Geometry check sheet. Reference: drawing and pictorial views, mm from the part's lowest x, y, z. A direction names the side the tool comes from. Give positions to 0.01 mm unless a question says otherwise; leave off trailing zeros. Loops run counter-clockwise (first coordinate to the right, second up) from the corner with the lowest first, then second, coordinate; pieces in that order, holes last. Notation, with made-up numbers: (76.5, -37.5) -> (94.5, -37.5) arc R25 cw to (94.5, 1.5) -> close; hole circle Ø7 at (86.25, 64). An arc over 180 degrees is marked (long way). Write item = value, one per line. Start each with the question number.
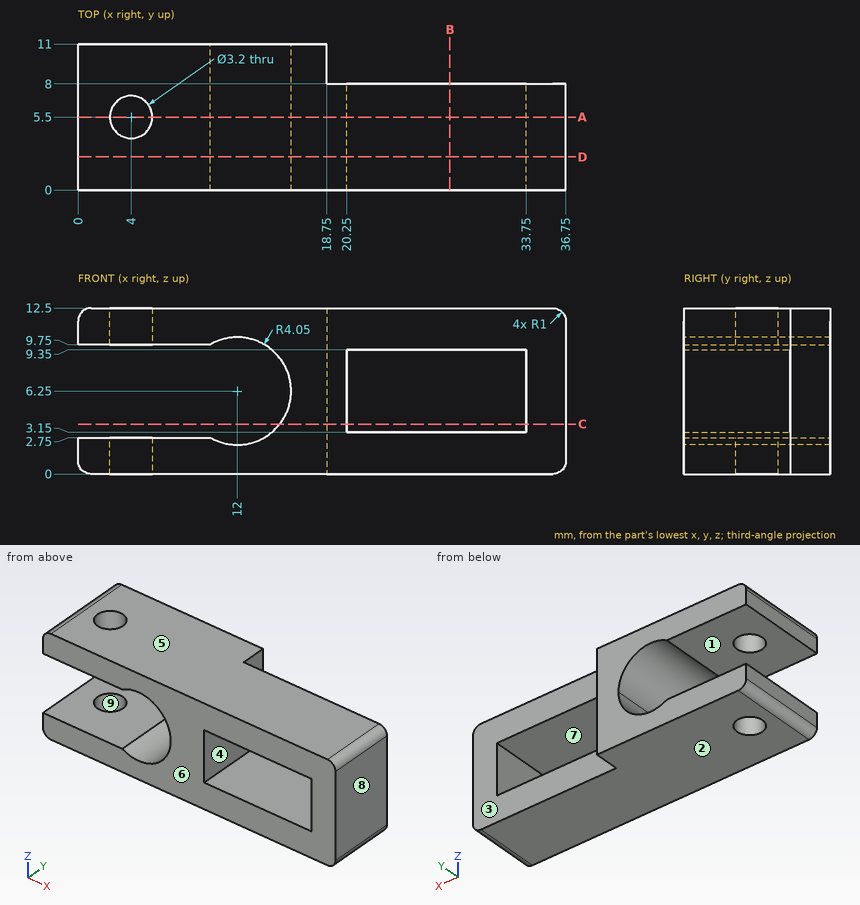
1) Draft check along X on the marked faces 6, 7, 8 and 9. Enter one of: released by +X, released by -X, zero draft, split by the parting line, or undercut.
2) Section check C-C (z = 3.75). Enter the section's corners in (x, y), plus the area to 3 significant figures.
3) Depth check by flat-ended pin: pin 1 Ø3 at (x, y) = (4, 5.5) entering from +Z; pin 2 Ø2.5 at (y, z) = (9.5, 3.5) entering from +X; pin 3 Ø3 at (y, z) = (3, 7) entering from -X. Enter the tip coordinate at first touch or a pass-through.
4) Thickness scan on line 1 (Y direction, x = 4, z = 11.5); line 2 (Z direction, x = 12, y = 8.5); line 3 (Z direction, x = 5, y = 2.75). Record the ranges inside material, lowest first.
5) Section check B-B (x = 28). Enter the section's corners in (y, z), plus the area to 3 significant figures.
6) Section check D-D (y = 2.5). Enter the section's corners in (x, z), plus the area to 3 significant figures.
7) Tool access check on the marked faces 1, 2, 3, 4 and 5. Record the directions out of +Z, -Z, +X, -X, +Y, -Y that give a thin tool (end or side, any length) a straight path to the whole face; none if there is none.
8) Section check A-A (y = 5.5). Enter the section's corners in (x, z).
Check result:
q1.face_6 = zero draft
q1.face_7 = undercut
q1.face_8 = released by +X
q1.face_9 = undercut
q2.outline = (15.19, 0) -> (20.25, 0) -> (20.25, 8) -> (18.75, 8) -> (18.75, 11) -> (15.19, 11) -> close; (33.75, 0) -> (36.75, 0) -> (36.75, 8) -> (33.75, 8) -> close
q2.area = 75.2 mm2
q3.pin_1 = through
q3.pin_2 = 18.75
q3.pin_3 = 15.37
q4.line_1 = 0 to 3.9, 7.1 to 11
q4.line_2 = 0 to 2.2, 10.3 to 12.5
q4.line_3 = 0 to 2.75, 9.75 to 12.5
q5.outline = (0, 0) -> (8, 0) -> (8, 3.15) -> (0, 3.15) -> close; (0, 9.35) -> (8, 9.35) -> (8, 12.5) -> (0, 12.5) -> close
q5.area = 50.4 mm2
q6.outline = (0, 1) arc R1 ccw to (1, 0) -> (35.75, 0) arc R1 ccw to (36.75, 1) -> (36.75, 11.5) arc R1 ccw to (35.75, 12.5) -> (1, 12.5) arc R1 ccw to (0, 11.5) -> (0, 9.75) -> (9.96, 9.75) arc R4.05 cw (long way) to (9.96, 2.75) -> (0, 2.75) -> close; hole (20.25, 3.15) -> (33.75, 3.15) -> (33.75, 9.35) -> (20.25, 9.35) -> close
q6.area = 264 mm2
q7.face_1 = -X, +Y, -Y
q7.face_2 = -Z, +X, -X, +Y, -Y
q7.face_3 = +Z, -Z, +X, +Y
q7.face_4 = +Y, -Y
q7.face_5 = +Z, +X, -X, +Y, -Y
q8.outline = (0, 1) arc R1 ccw to (1, 0) -> (2.4, 0) -> (2.4, 2.75) -> (0, 2.75) -> close; (0, 9.75) -> (2.4, 9.75) -> (2.4, 12.5) -> (1, 12.5) arc R1 ccw to (0, 11.5) -> close; (5.6, 0) -> (35.75, 0) arc R1 ccw to (36.75, 1) -> (36.75, 11.5) arc R1 ccw to (35.75, 12.5) -> (5.6, 12.5) -> (5.6, 9.75) -> (9.96, 9.75) arc R4.05 cw (long way) to (9.96, 2.75) -> (5.6, 2.75) -> close; hole (20.25, 3.15) -> (33.75, 3.15) -> (33.75, 9.35) -> (20.25, 9.35) -> close
